The model under review builds one solid part; all positions refer to its coordinate system, in mm. A direction names the side the tool comes from. Give positions to 0.01 mm unless a question says otherwise; leave off trailing zeros. Order: outer loops, then holes, each group sorted by start corner. A loop starts at its lowest first (then second) coordinate and runs counter-clockwise, first axis right, second up. Notation, with made-up numbers: (14.5, -23.5) - (56.5, -23.5) arc R16 ccw to (56.5, 2.5) - close; hole circle Ø4 at (-27.75, 33.5). An arc over 180 degrees is marked (long way). Use a Markdown table: item, result. Add a question column.
```python
from build123d import *

# Parameters (mm, degrees)
F0_W     = 19.05
F0_H     = 254
F1_DEPTH = 254
F2_W     = 19.05
F2_H     = 38.1
F3_DEPTH = 19.05
F4_W     = 19.05
F4_H     = 38.1
F5_DEPTH = 19.05
F6_W     = 19.05
F6_H     = 38.1
F7_DEPTH = 19.05


with BuildPart() as f1:
    # F0 (on Top) → F1 (new body)
    with BuildSketch(Plane.XY):
        with Locations((47.761202, 2.701772)):
            Rectangle(F0_W, F0_H)
    extrude(amount=F1_DEPTH)

    # F2 (on face) → F3 (join)
    with BuildSketch(Plane.XZ.offset(124.298228)):
        with Locations((47.761202, 76.2)):
            Rectangle(F2_W, F2_H)
        with Locations((47.761202, 177.8)):
            Rectangle(F2_W, F2_H)
    extrude(amount=F3_DEPTH)

    # F4 (on face) → F5 (join)
    with BuildSketch(Plane.XY.offset(254)):
        with Locations((47.761202, 53.501772)):
            Rectangle(F4_W, F4_H)
        with Locations((47.761202, -48.098228)):
            Rectangle(F4_W, F4_H)
    extrude(amount=F5_DEPTH)

    # F6 (on face) → F7 (join)
    with BuildSketch(Plane(origin=(0, 129.701772, 0), x_dir=(-1, 0, 0), z_dir=(0, 1, 0))):
        with Locations((-47.761202, 76.2)):
            Rectangle(F6_W, F6_H)
        with Locations((-47.761202, 177.8)):
            Rectangle(F6_W, F6_H)
    extrude(amount=F7_DEPTH)


solid = f1.part
```
Q1. We need section B-B (z = 233). Write out the cut boundary in (x, y).
Q2. We need section A-A (x = 48.75). Write out the cut boundary in (y, z), plus the area to 3 significant figures.
Q3. We need section C-C (y = 106.5). Write out the cut boundary in (x, z).
Q4. Wall thickness on probe 1 along Z at (x, y) = (49, 82); probe 2 along Y at (x, z) = (39, 103.5): over which ranges is each line inside the solid? List them lowest first.
Q5. Draft analysis for pull direction Z (two halves, no side actions). For faces 1 (the flat face through (48, 139, 158.75)), 2 (the flat face through (48, -67.148, 263)), 3 (the flat face through (48, -134, 57.15)), state which applies: pulls with the +Z half, pulls with the -Z half, needs draft (parallel to the pull), parting line crosses it, or undercut.
Q6. Machinability: for faces 4 (the flat face through (48, -124.298, 28)), 5 (the flat face through (48, 129.702, 225)), 6 (the flat face through (48, 139, 95.25)), 7 (the flat face through (48, -124.298, 225)), 8 (the flat face through (48, -29.048, 263)), which of the approach directions +Z, -Z, +X, -X, +Y, -Y give a long, thin tool a straight path to every point of the face, cutting with its end or side? Answer none if there is none.
Q7. Clearance check with flat-ended pins moving along their axes: P1, Ø9.5, axis at x = 43, y = 138.5, coming from the -Z side; P2, Ø5.5, axis at x = 48.5, y = 143, coming from the +Z side; P3, Ø2, axis at x = 53.5, z = 123.5, coming from the +Y side. State where each tip first meets the part, or that it passes through.
Here are the results:
| question | item | result |
|---|---|---|
| 1 | outline | (38.24, -124.3) - (57.29, -124.3) - (57.29, 129.7) - (38.24, 129.7) - close |
| 2 | outline | (-143.35, 57.15) - (-124.3, 57.15) - (-124.3, 0) - (129.7, 0) - (129.7, 57.15) - (148.75, 57.15) - (148.75, 95.25) - (129.7, 95.25) - (129.7, 158.75) - (148.75, 158.75) - (148.75, 196.85) - (129.7, 196.85) - (129.7, 254) - (72.55, 254) - (72.55, 273.05) - (34.45, 273.05) - (34.45, 254) - (-29.05, 254) - (-29.05, 273.05) - (-67.15, 273.05) - (-67.15, 254) - (-124.3, 254) - (-124.3, 196.85) - (-143.35, 196.85) - (-143.35, 158.75) - (-124.3, 158.75) - (-124.3, 95.25) - (-143.35, 95.25) - close |
| 2 | area | 68,900 mm2 |
| 3 | outline | (38.24, 0) - (57.29, 0) - (57.29, 254) - (38.24, 254) - close |
| 4 | probe 1 | 0 to 254 |
| 4 | probe 2 | -124.3 to 129.7 |
| 5 | face 1 | undercut |
| 5 | face 2 | needs draft |
| 5 | face 3 | pulls with the -Z half |
| 6 | face 4 | -Z, +X, -X, -Y |
| 6 | face 5 | +Z, +X, -X, +Y |
| 6 | face 6 | +X, -X, +Y |
| 6 | face 7 | +Z, +X, -X, -Y |
| 6 | face 8 | +Z, +X, -X |
| 7 | P1 | z = 57.15 |
| 7 | P2 | z = 196.85 |
| 7 | P3 | y = 129.7 |
